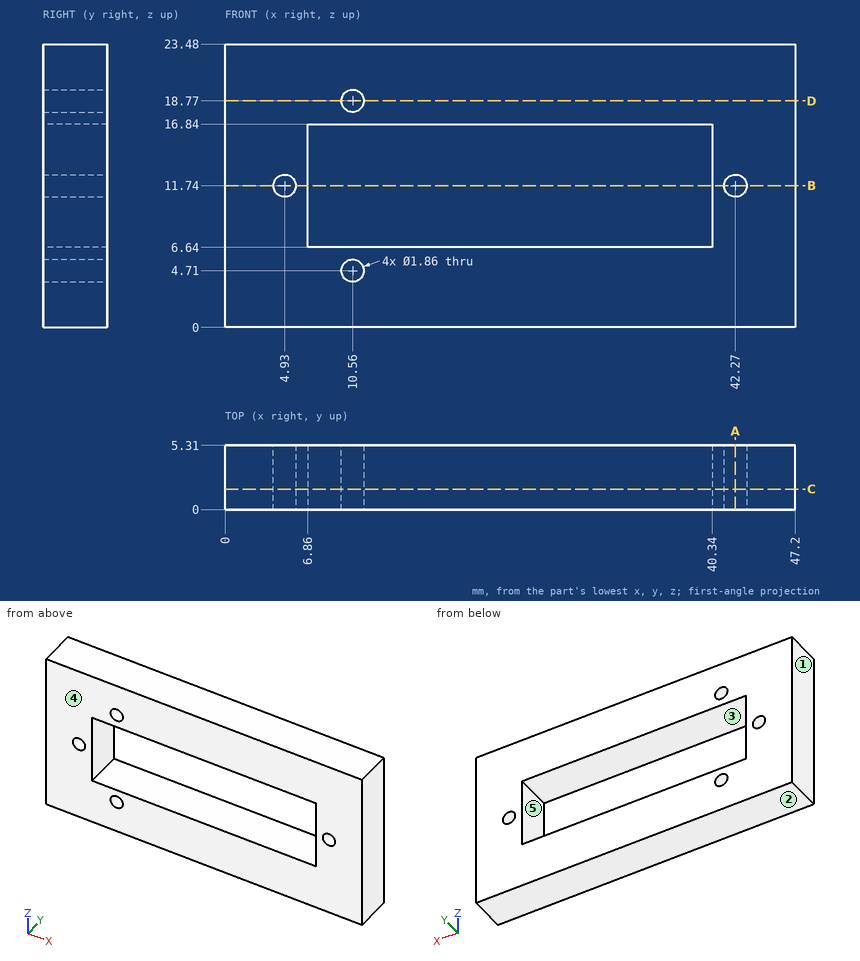
The drawing under review shows one solid part. Ordinate dimensions are in mm from its lowest x, y, z. A direction names the side the tool comes from. Coordinates: 2 decimals unless noted, no trailing zeros. Write each loop counter-clockwise with the first axis right and the second up, starting at its lowest first coordinate (ties: lowest second). Pieces come first, ordered by that corner, then holes. Notation, with made-up numbers: M 60.25,89 L 103.25,89 A21 cw 103.25,121 Z; hole C -2,81.5 d2. An arc over 180 degrees is marked long. Put each result on its own line as item: value.
1) Draft analysis for pull direction Z (two halves, no side actions). For the marked faces 1, 2 and 3, state which applies: released by +Z, released by -Z, zero draft, split by the parting line, or undercut.
Computed:
face 1: zero draft
face 2: released by -Z
face 3: undercut
2) Add section C-C on y = 1.7. Give the boundary of the cut face in (x, z), then the cut area to 3 significant figures.
Computed:
outline: M 0,0 L 47.2,0 L 47.2,23.48 L 0,23.48 Z; hole C 4.93,11.74 d1.86; hole M 6.86,6.64 L 40.34,6.64 L 40.34,16.84 L 6.86,16.84 Z; hole C 10.56,4.71 d1.86; hole C 10.56,18.77 d1.86; hole C 42.27,11.74 d1.86
area: 756 mm2
3) Clearance check with a flat-ended pin moving along its axis: pin 1 Ø1.5 at (x, z) = (4.93, 11.74) entering from -Y. State where the tip first meets the part, or that it passes through.
Computed:
pin 1: passes through
4) Add section A-A on x = 42.27. Give the boundary of the cut face in (y, z), then the cut area to 3 significant figures.
Computed:
outline: M 0,0 L 5.31,0 L 5.31,10.81 L 0,10.81 Z; M 0,12.67 L 5.31,12.67 L 5.31,23.48 L 0,23.48 Z
area: 115 mm2
5) Add section B-B on z = 11.74. Give the boundary of the cut face in (x, y).
Computed:
outline: M 0,0 L 4,0 L 4,5.31 L 0,5.31 Z; M 5.86,0 L 6.86,0 L 6.86,5.31 L 5.86,5.31 Z; M 40.34,0 L 41.34,0 L 41.34,5.31 L 40.34,5.31 Z; M 43.2,0 L 47.2,0 L 47.2,5.31 L 43.2,5.31 Z
6) For the marked faces 4 and 5, list the 3-axis set-ups (+Z, -Z, +X, -X, +Y, -Y) from which the entire face can be reached by the end or side of a thin tool; tool diameter is ignored.
Computed:
face 4: +Z, -Z, +X, -X, -Y
face 5: +Y, -Y
7) Wall thickness on probe 1 along X at (y, z) = (1.35, 11.74); probe 2 along X at (y, z) = (4.5, 9.5); probe 3 along Z at (x, y) = (36.5, 4.2): over which ranges is each line inside the solid? List them lowest first. Write a range as [from, to].
Computed:
probe 1: x = [0, 4], [5.86, 6.86], [40.34, 41.34], [43.2, 47.2]
probe 2: x = [0, 6.86], [40.34, 47.2]
probe 3: z = [0, 6.64], [16.84, 23.48]
8) Add section D-D on z = 18.77. Give the boundary of the cut face in (x, y), then the cut area to 3 significant figures.
Computed:
outline: M 0,0 L 9.63,0 L 9.63,5.31 L 0,5.31 Z; M 11.49,0 L 47.2,0 L 47.2,5.31 L 11.49,5.31 Z
area: 241 mm2
